Part model, mm, in its own coordinate system. Face numbers are marked on the shaded views. A direction names the side the tool comes from. Give positions to 0.01 mm unless a question says otherwise; leave off trailing zeros. Order: outer loops, then holes, each group sorted by start corner. A loop starts at its lowest first (then second) coordinate and runs counter-clockwise, first axis right, second up. Notation, with made-up numbers: (75.5, 27) - (85.5, 27) arc R23 ccw to (85.5, 62) - close; hole circle Ø2 at (-33, 72). An arc over 180 degrees is marked (long way). One line per item, written item: value.
```python
from build123d import *

# Parameters (mm, degrees)
CYLINDER003_R     = 3.5
CYLINDER003_DEPTH = 62
ARRAY_Z_COUNT     = 5
ARRAY_Z_PITCH     = 5
CYLINDER001_R     = 7
CYLINDER001_DEPTH = 5
CYLINDER002_R     = 9.5
CYLINDER002_DEPTH = 3.559183
CYLINDER004_R     = 4
CYLINDER004_DEPTH = 62
CYLINDER_R        = 6
CYLINDER_DEPTH    = 60
TORUS_R           = 2


with BuildPart() as cylinder003:
    # Cylinder003 → Cylinder003 (new body)
    with BuildSketch(Plane.XY):
        Circle(CYLINDER003_R)
    extrude(amount=CYLINDER003_DEPTH)


with BuildPart() as fusion002:
    # Cone → Cone (revolve)
    with BuildSketch(Plane.XZ):
        Polygon((0, 0), (7, 0), (6, 8), (0, 8), align=None)
    revolve(axis=Axis((0, 0, 0), (0, 0, 1)))

    # Array Z: Fusion002 ×5


with BuildPart() as fusion002_1:
    add(fusion002.part)
    with Locations(*[(0, 0, i * ARRAY_Z_PITCH) for i in range(1, ARRAY_Z_COUNT)]):
        add(fusion002.part)


with BuildPart() as fusion002_2:
    # Array placement: moved
    add(fusion002_1.part.moved(Location((0, 0, 15))))


with BuildPart() as cylinder001:
    # Cylinder001 → Cylinder001 (new body)
    with BuildSketch(Plane.XY.offset(10)):
        Circle(CYLINDER001_R)
    extrude(amount=CYLINDER001_DEPTH)


with BuildPart() as cylinder002:
    # Cylinder002 → Cylinder002 (new body)
    with BuildSketch(Plane.XY.offset(6.440817)):
        Circle(CYLINDER002_R)
    extrude(amount=CYLINDER002_DEPTH)


with BuildPart() as fusion:
    # Cone001 → Cone001 (revolve)
    with BuildSketch(Plane(origin=(0, 0, 6), x_dir=(1, 0, 0), z_dir=(0, -1, 0))):
        Polygon((0, 0), (6, 0), (9.5, 0.440817), (0, 0.440817), align=None)
    revolve(axis=Axis((0, 0, 6), (0, 0, 1)))

    # Fusion: union Cylinder001, Cylinder002
    add(cylinder001.part)
    add(cylinder002.part)


with BuildPart() as cylinder004:
    # Cylinder004 → Cylinder004 (new body)
    with BuildSketch(Plane.XY):
        Circle(CYLINDER004_R)
    extrude(amount=CYLINDER004_DEPTH)


with BuildPart() as fusion003:
    # Cylinder → Cylinder (new body)
    with BuildSketch(Plane.XY):
        Circle(CYLINDER_R)
    extrude(amount=CYLINDER_DEPTH)

    # Fusion001: union Fusion, Cylinder004
    add(fusion.part)
    add(cylinder004.part)

    # Fusion003: union Fusion002
    add(fusion002_2.part)


with BuildPart() as obj1:
    # Torus → Torus (revolve)
    with BuildSketch(Plane(origin=(0, 0, 60), x_dir=(1, 0, 0), z_dir=(0, -1, 0))):
        with Locations((4, 0)):
            Circle(TORUS_R)
    revolve(axis=Axis((0, 0, 60), (0, 0, 1)))

    # Fusion004: union Fusion003
    add(fusion003.part)

    # Cut: cut Cylinder003
    add(cylinder003.part, mode=Mode.SUBTRACT)


solid = obj1.part
```
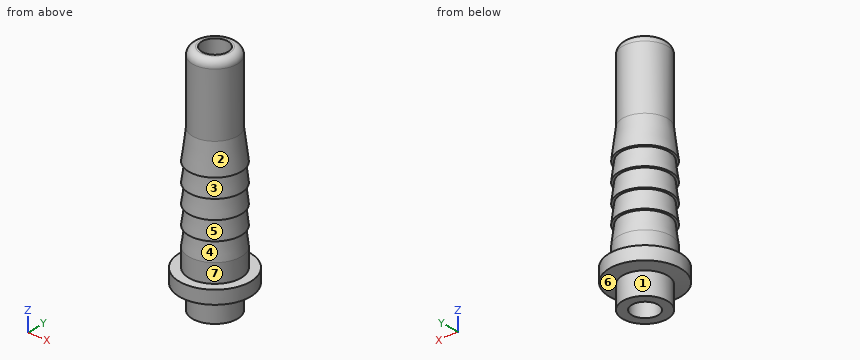
1) Drop flat-ended pins along their axis: P1, Ø8, axis at x = 2, z = 55.5, coming from the -Y side; P2, Ø10, axis at x = 7.5, z = 20.5, coming from the -Y side; P3, Ø1, axis at x = 3, y = -4, coming from the +Z side. Give the stop position or say it passes through.
Answer:
P1: stops at y = -6
P2: stops at y = -6.53
P3: stops at z = 61.94
2) Slice it at A-A on z = 37. Write the cut outline in (x, y), then the cut area to 3 significant figures.
Answer:
outline: circle Ø13.5 at (0, 0); hole circle Ø7 at (0, 0)
area: 105 mm2
3) Which spindle directions (+Z, -Z, +X, -X, +Y, -Y) get a long thin tool onto all of the face, cutting with end or side? Do the marked faces 5, 6 and 7. Say none if no direction does.
Answer:
face 5: none
face 6: -Z
face 7: +Z
4) Two-plate mould, pull along Z, no slides. Class the marked faces 1, 2, 3 and 4: pulls with the +Z half, pulls with the -Z half, needs draft (parallel to the pull), parting line crosses it, or undercut.
Answer:
face 1: needs draft
face 2: pulls with the +Z half
face 3: undercut
face 4: undercut
5) Slice it at B-B on z = 54. Write the cut outline in (x, y), then the cut area to 3 significant figures.
Answer:
outline: circle Ø12 at (0, 0); hole circle Ø7 at (0, 0)
area: 74.6 mm2
6) Wall check: line 1 along X through (y, z) = (0.25, 11.5); line 2 along X through (y, z) = (-2, 49); line 3 along Y through (x, z) = (0, 36) (3 decimals). Give the ranges that are in metal, low to high. Write a range as [from, to].
Answer:
line 1: x = [-7, -3.49], [3.49, 7]
line 2: x = [-5.66, -2.87], [2.87, 5.66]
line 3: y = [-6.875, -3.5], [3.5, 6.875]
